Can you work these out from the drawing? Everything is in mm from the part's minimum corner. A direction names the side the tool comes from. Coordinates: 2 decimals unless noted, no trailing zeros. Order: outer loops, then holes, each group sorted by start corner. A loop starts at its lowest first (then second) coordinate and runs counter-clockwise, first axis right, second up. Notation, with made-up numbers: (47.5, 55.5) - (67.5, 55.5) arc R24 ccw to (67.5, 93.5) - close; hole circle Ø6 at (82, 39). An arc over 180 degrees is marked (long way). Answer as CSV lines item,"result". Start each with the question number.
Item 1: Imagine slicing it at B-B on y = 15. List the corners of the cut face in (x, z) for me.
Item 2: I'm going to push flat-ended pins straight in: pin 1 (3.5 mm diameter, centred on y = 3, z = 4, fed in from +X); pin 2 (5 mm diameter, centred on x = 4.5, z = 6, fed in from +Y); pin 3 (1.2 mm diameter, centred on y = 3.5, z = 5, fed in from -X); pin 4 (3 mm diameter, centred on x = 5.5, z = 6, fed in from -Y). Where does each tip first touch, or does it pass through?
Item 3: Imagine slicing it at C-C on y = 7. List the corners of the cut face in (x, z) for me, and give its area (3 significant figures).
Item 4: Imagine slicing it at A-A on z = 2.25. List the corners of the cut face in (x, y) for me, and give its area (3 significant figures).
Item 5: I need wall thicknesses on line 1 (X direction, y = 12.75, z = 4); line 2 (Y direction, x = 6, z = 0.5); line 3 (X direction, y = 3.5, z = 9.25). Which ranges of each line are inside material? Lowest first, please.
Item 6: On a 3-axis mill with a long thin cutter (end or side, diameter ignored), from which of +Z, -Z, +X, -X, +Y, -Y can I reach the whole of each face in a straight line? I mean the marked faces 1, 2 and 3. Say none if no direction works.
Item 7: Imagine slicing it at D-D on x = 13. List the corners of the cut face in (y, z) for me.
Item 8: We'd pull the mould along Y, two halves only. Please class the marked faces 4, 5 and 6: pulls with the +Y half, pulls with the -Y half, needs draft (parallel to the pull), parting line crosses it, or undercut.
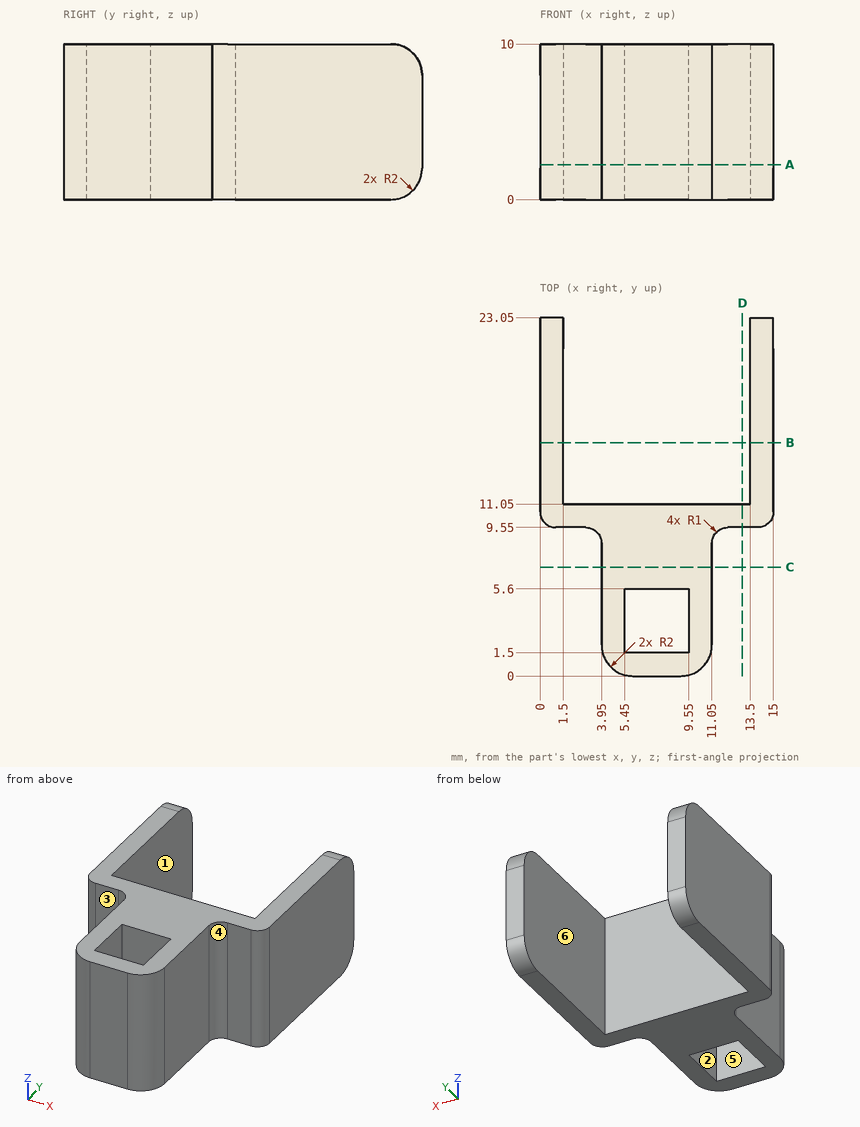
Responses:
1,outline,"(0, 0) - (1.5, 0) - (1.5, 10) - (0, 10) - close; (13.5, 0) - (15, 0) - (15, 10) - (13.5, 10) - close"
2,pin 1,"stops at x = 11.05"
2,pin 2,"stops at y = 11.05"
2,pin 3,"stops at x = 3.95"
2,pin 4,"stops at y = 0"
3,outline,"(3.95, 0) - (11.05, 0) - (11.05, 10) - (3.95, 10) - close"
3,area,"71.0 mm^2"
4,outline,"(0, 10.55) arc R1 ccw to (1, 9.55) - (2.95, 9.55) arc R1 cw to (3.95, 8.55) - (3.95, 2) arc R2 ccw to (5.95, 0) - (9.05, 0) arc R2 ccw to (11.05, 2) - (11.05, 8.55) arc R1 cw to (12.05, 9.55) - (14, 9.55) arc R1 ccw to (15, 10.55) - (15, 23.05) - (13.5, 23.05) - (13.5, 11.05) - (1.5, 11.05) - (1.5, 23.05) - (0, 23.05) - close; hole (5.45, 1.5) - (9.55, 1.5) - (9.55, 5.6) - (5.45, 5.6) - close"
4,area,"108 mm^2"
5,line 1,"x = 0 to 1.5, 13.5 to 15"
5,line 2,"y = 0 to 1.5, 5.6 to 11.05"
5,line 3,"x = 3.95 to 5.45, 9.55 to 11.05"
6,face 1,"+Z, -Z, +Y"
6,face 2,"+Z, -Z"
6,face 3,"+Z, -Z, -X, -Y"
7,outline,"(9.55, 0) - (11.05, 0) - (11.05, 10) - (9.55, 10) - close"
8,face 4,"pulls with the -Y half"
8,face 5,"undercut"
8,face 6,"needs draft"
